Design review of the part built by this model. Coordinates are the model's own, in mm. A direction names the side the tool comes from. Coordinates: 2 decimals unless noted, no trailing zeros. Loops run counter-clockwise (first coordinate to the right, second up) from the corner with the lowest first, then second, coordinate; pieces in that order, holes last. Notation, with made-up numbers: (32.5, 73) -> (80.5, 73) arc R28 cw to (80.5, 103) -> close; hole circle Ø11 at (89.25, -18). An arc over 180 degrees is marked (long way). Use CSV: the item, a comma, the result in double quotes.
```python
from build123d import *

# Parameters (mm, degrees)
SKETCH_1_R      = 1.45
EXTRUDE_1_DEPTH = 2
FILLET_2_R      = 3
FILLET_3_R      = 2


with BuildPart() as part:
    # 草图1 → 凸台-拉伸1 (new body)
    with BuildSketch(Plane(origin=(0, 0, 0), x_dir=(1, 0, 0), z_dir=(0, 1, 0))):
        Polygon((-7.5, 27.5), (-22.5, 7.5), (-22.5, -7.5), (22.5, -7.5), (22.5, 7.5), (7.5, 27.5), align=None)
        with Locations(Location((-17.5, 0, 0), (0, 0, 270))):
            Circle(SKETCH_1_R, mode=Mode.SUBTRACT)
        with Locations(Location((17.5, 0, 0), (0, 0, 270))):
            Circle(SKETCH_1_R, mode=Mode.SUBTRACT)
        with Locations(Location((0, 12.5, 0), (0, 0, 270))):
            Circle(SKETCH_1_R, mode=Mode.SUBTRACT)
        with Locations(Location((0, 22.5, 0), (0, 0, 270))):
            Circle(SKETCH_1_R, mode=Mode.SUBTRACT)
        Polygon((-7.5, 22.5), (-18.75, 7.5), (-7.5, 7.5), align=None, mode=Mode.SUBTRACT)
        Polygon((18.75, 7.5), (7.5, 7.5), (7.5, 22.5), align=None, mode=Mode.SUBTRACT)
    extrude(amount=EXTRUDE_1_DEPTH)

    # 圆角2
    fillet_2_edges = [part.edges().sort_by_distance(p)[0] for p in [
        (22.5, 1, -7.5),
        (22.5, 1, 7.5),
        (-22.5, 1, 7.5),
        (-22.5, 1, -7.5),
        (-7.5, 1, -27.5),
        (7.5, 1, -27.5),
    ]]
    fillet(fillet_2_edges, radius=FILLET_2_R)

    # 圆角3
    fillet_3_edges = [part.edges().sort_by_distance(p)[0] for p in [
        (-7.5, 1, -7.5),
        (-7.5, 1, -22.5),
        (-18.75, 1, -7.5),
        (18.75, 1, -7.5),
        (7.5, 1, -22.5),
        (7.5, 1, -7.5),
    ]]
    fillet(fillet_3_edges, radius=FILLET_3_R)


solid = part.part
```
Item 1: Machinability: for faces 1 (the face through (7.5, 1, -13)), 2 (the face through (-22.5, 1, -1)), which of the approach directions +Z, -Z, +X, -X, +Y, -Y give a long, thin tool a straight path to every point of the face, cutting with its end or side? Answer none if there is none.
Checked values:
face 1,"+Y, -Y"
face 2,"+Z, -Z, -X, +Y, -Y"
Item 2: To check wall thickness, follow line 1 along X through (y, z) = (0.6, 0); line 2 along X through (y, z) = (0.7, -14) (3 decimals); line 3 along X through (y, z) = (0.75, -12.5). State the ranges of each line that lie inside material, in increasing order.
Checked values:
line 1,"-22.5 to -18.95, -16.05 to 16.05, 18.95 to 22.5"
line 2,"-17.625 to -13.875, -7.5 to 7.5, 13.875 to 17.625"
line 3,"-18.75 to -15, -7.5 to -1.45, 1.45 to 7.5, 15 to 18.75"
Item 3: Add section A-A (z = 0). Give the boundary of the cut face in (x, y).
Checked values:
outline,"(-22.5, 0) -> (-18.95, 0) -> (-18.95, 2) -> (-22.5, 2) -> close; (-16.05, 0) -> (16.05, 0) -> (16.05, 2) -> (-16.05, 2) -> close; (18.95, 0) -> (22.5, 0) -> (22.5, 2) -> (18.95, 2) -> close"
Item 4: Add section D-D (z = -12.5). Give the boundary of the cut face in (x, y).
Checked values:
outline,"(-18.75, 0) -> (-15, 0) -> (-15, 2) -> (-18.75, 2) -> close; (-7.5, 0) -> (-1.45, 0) -> (-1.45, 2) -> (-7.5, 2) -> close; (1.45, 0) -> (7.5, 0) -> (7.5, 2) -> (1.45, 2) -> close; (15, 0) -> (18.75, 0) -> (18.75, 2) -> (15, 2) -> close"
Item 5: Add section B-B (y = 0.55). Give the boundary of the cut face in (x, z), then the cut area to 3 significant figures.
Checked values:
outline,"(-22.5, -6.5) arc R3 ccw to (-21.9, -8.3) -> (-8.4, -26.3) arc R3 ccw to (-6, -27.5) -> (6, -27.5) arc R3 ccw to (8.4, -26.3) -> (21.9, -8.3) arc R3 ccw to (22.5, -6.5) -> (22.5, 4.5) arc R3 ccw to (19.5, 7.5) -> (-19.5, 7.5) arc R3 ccw to (-22.5, 4.5) -> close; hole circle Ø2.9 at (-17.5, 0); hole (-16.35, -10.7) -> (-11.1, -17.7) arc R2 ccw to (-7.5, -16.5) -> (-7.5, -9.5) arc R2 ccw to (-9.5, -7.5) -> (-14.75, -7.5) arc R2 ccw to start; hole circle Ø2.9 at (0, -22.5); hole circle Ø2.9 at (0, -12.5); hole (7.5, -16.5) arc R2 ccw to (11.1, -17.7) -> (16.35, -10.7) arc R2 ccw to (14.75, -7.5) -> (9.5, -7.5) arc R2 ccw to (7.5, -9.5) -> close; hole circle Ø2.9 at (17.5, 0)"
area,"1,100 mm^2"
Item 6: Add section C-C (x = 17.5). Give the boundary of the cut face in (y, z), then the cut area to 3 significant figures.
Checked values:
outline,"(0, -14.17) -> (2, -14.17) -> (2, -1.45) -> (0, -1.45) -> close; (0, 1.45) -> (2, 1.45) -> (2, 7.5) -> (0, 7.5) -> close"
area,"37.5 mm^2"
Item 7: Draft analysis for pull direction X (two halves, no side actions). For faces 3 (the face through (-21.64, 1.01, 6.6)), 4 (the face through (7.324, 1.014, -27.192)), 5 (the face through (8.901, 1.014, -18.408)), state which applies: pulls with the +X half, pulls with the -X half, needs draft (parallel to the pull), parting line crosses it, or undercut.
Checked values:
face 3,"pulls with the -X half"
face 4,"pulls with the +X half"
face 5,"undercut"
